from build123d import *

# Parameters (mm, degrees)
SKETCH2_R               = 6.25
CUT_EXTRUDE1_DEPTH      = 26.0000001
CUT_EXTRUDE1_DEPTH_BACK = 26.0000001
BOSS_EXTRUDE4_START     = 12.5
SKETCH3_R               = 7.25
SKETCH3_R_2             = 6.25
BOSS_EXTRUDE4_DEPTH     = 11.425666


with BuildPart() as part:
    # Sketch1 → Revolve1 (revolve)
    with BuildSketch(Plane.XY):
        with BuildLine():
            Line((23, 0), (25, 0))
            Line((25, 0), (25, 41.5))
            Line((25, 41.5), (22.5, 41.5))
            Line((22.5, 41.5), (22.5, 44))
            Line((22.5, 44), (25, 44))
            Line((25, 44), (25, 47))
            Line((25, 47), (22.5, 47))
            Line((22.5, 47), (22.5, 49.5))
            Line((22.5, 49.5), (25, 49.5))
            Line((25, 49.5), (25, 54.5))
            ThreePointArc((25, 54.5), (13.174901691, 60.609067785), (0, 62.5))
            Line((0, 62.5), (0, 60.49936285))
            ThreePointArc((0, 60.49936285), (12.069492637, 58.859165445), (23, 53.484511145))
            Line((23, 53.484511145), (23, 51.5))
            Line((23, 51.5), (20.5, 51.5))
            Line((20.5, 51.5), (20.5, 39.5))
            Line((20.5, 39.5), (23, 39.5))
            Line((23, 39.5), (23, 0))
        make_face()
    revolve(axis=Axis((0, 62.5, 0), (0, -1, 0)))

    # Sketch2 → Cut-Extrude1 (cut, two sides)
    with BuildSketch(Plane.XY) as cut_extrude1_sk:
        with Locations((0, 30.5)):
            Circle(SKETCH2_R)
        with BuildLine():
            ThreePointArc((16.733200531, 0), (0, 10), (-16.733200531, 0))
            Line((-16.733200531, 0), (16.733200531, 0))
        make_face()
    extrude(amount=CUT_EXTRUDE1_DEPTH, mode=Mode.SUBTRACT)
    extrude(cut_extrude1_sk.sketch, amount=-CUT_EXTRUDE1_DEPTH_BACK, mode=Mode.SUBTRACT)

    # Sketch3 → Boss-Extrude4 (add)
    with BuildSketch(Plane.XY.offset(BOSS_EXTRUDE4_START)):
        with Locations((0, 30.5)):
            Circle(SKETCH3_R)
        with Locations((0, 30.5)):
            Circle(SKETCH3_R_2, mode=Mode.SUBTRACT)
    boss_extrude4 = extrude(amount=BOSS_EXTRUDE4_DEPTH)

    # Mirror1: Boss-Extrude4 across plane
    add(boss_extrude4.mirror(Plane.XY))


solid = part.part
Work out the finished part from the listing and answer in its coordinate system (mm). A direction names the side the tool comes from. Round coordinates to 2 decimals unless told otherwise and drop trailing zeros. Write each loop counter-clockwise with the first axis right and the second up, starting at its lowest first coordinate (ties: lowest second). Pieces come first, ordered by that corner, then holes. Notation, with made-up numbers: (31, 89.25) - (74, 89.25) arc R6 ccw to (74, 98.25) - close; hole circle Ø1 at (26, 66.5). An arc over 180 degrees is marked (long way). Answer in a Markdown table with one row per item. Add a question column.
1. For faces 1 (the flat face through (23.3, 0, 0.1)), 2 (the flat face through (-6, 33, -12.5)), 3 (the cylindrical face through (10.382, 42.768, -19.961)), determine the directions among +Z, -Z, +X, -X, +Y, -Y from which every point of the face is accessible in a straight line to the end or side of a thin tool.
2. A cutting plane is placed at B-B, the plane z = -17. Count the separate pieces of the cut face and the enclosed holes in it, and give its area (3 significant figures).
3. A cutting plane is placed at C-C, the plane y = 52.5. Determine the outline of the cut face in (x, z).
4. A cutting plane is placed at A-A, the plane y = 30.5. Determine the outline of the cut face in (x, z).
5. The mould has two halves that part along Z. Classify faces 4 (the cylindrical face through (-0.94, 37.69, 17.69)), 5 (the flat face through (22.34, 49.5, 3.82)), 6 (the cylindrical face through (10.382, 48.268, -19.961)): +Z half, -Z half, draft (parallel to the pull), parting line (faces both ways), or undercut.
6. Given pin 1 (11.5 mm diameter, centred on x = -2.5, y = 31, fed in from -Z); pin 2 (5 mm diameter, centred on y = 31, z = -4, fed in from -X); pin 3 (12 mm diameter, centred on x = -9.5, y = 49, fed in from +Z), each flat-ended and moving along its own axis, determine where each tip first touches the part or whether it passes through.
7. Find the intervals of material crossed by line 1 along X through (y, z) = (30, 16); line 2 along Y through (x, z) = (2, 14); line 3 along Z through (x, y) = (0, 52.2), in increasing order. Write a range as from..to.
Worked out:
| question | item | result |
|---|---|---|
| 1 | face 1 | +Z, -Z, +X, -X, -Y |
| 1 | face 2 | -Y |
| 1 | face 3 | none |
| 2 | separate pieces | 2 |
| 2 | enclosed holes | 1 |
| 2 | area | 484 mm^2 |
| 3 | outline | circle Ø50 at (0, 0); hole circle Ø46 at (0, 0) |
| 4 | outline | (-7.25, -21.83) arc R23 cw to (-7.25, 21.83) - (-7.25, 12.5) - (-6.25, 12.5) - (-6.25, 24.21) arc R25 ccw to (-6.25, -24.21) - (-6.25, -12.5) - (-7.25, -12.5) - close; (6.25, -24.21) arc R25 ccw to (6.25, 24.21) - (6.25, 12.5) - (7.25, 12.5) - (7.25, 21.83) arc R23 cw to (7.25, -21.83) - (7.25, -12.5) - (6.25, -12.5) - close |
| 5 | face 4 | undercut |
| 5 | face 5 | draft |
| 5 | face 6 | parting line |
| 6 | pin 1 | z = -24.97 |
| 6 | pin 2 | x = -24.95 |
| 6 | pin 3 | z = 24.75 |
| 7 | line 1 | -19.21..-16.52, -7.23..-6.23, 6.23..7.23, 16.52..19.21 |
| 7 | line 2 | 23.53..24.58, 36.42..37.47, 58.16..60.29 |
| 7 | line 3 | -25..-23, 23..25 |
